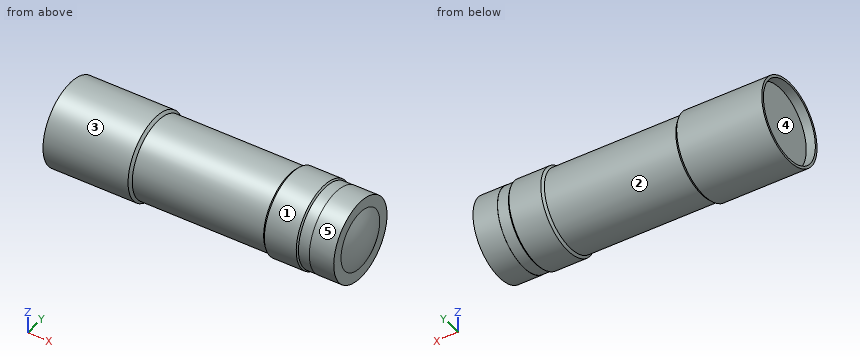
```python
from build123d import *

# Parameters (mm, degrees)
F2_SIZE = 0.74999
F3_SIZE = 0.64999
F4_SIZE = 0.39999


# Not quite as in the source:
# - a fillet or chamfer is up to 0.001 mm smaller than in the source, because OpenCascade refuses the exact size


with BuildPart() as f1:
    # F0 (on Front) → F1 (revolve)
    with BuildSketch(Plane.XZ):
        with BuildLine():
            Line((-85.55, 11.75), (-85.55, 0))
            Line((-85.55, 0), (0, 0))
            ThreePointArc((0, 0), (-0.5715031948, 4.5173277499), (-2.25, 8.75))
            Line((-2.25, 8.75), (-2.25, 12.05))
            Line((-2.25, 12.05), (-9.5, 12.05))
            Line((-9.5, 12.05), (-9.5, 12))
            Line((-9.5, 12), (-12.75, 12))
            Line((-12.75, 12), (-12.75, 12.4))
            Line((-12.75, 12.4), (-23.25, 12.4))
            Line((-23.25, 12.4), (-23.25, 11.75))
            Line((-23.25, 11.75), (-62.25, 11.75))
            Line((-62.25, 11.75), (-62.25, 12.5))
            Line((-62.25, 12.5), (-88.25, 12.5))
            Line((-88.25, 12.5), (-88.25, 11.75))
            Line((-88.25, 11.75), (-85.55, 11.75))
        make_face()
    revolve(axis=Axis((-46.3619604707, 0, 0), (-1, 0, 0)))

    # F2 (size 0.75 in the source; OpenCascade refuses exactly that, so slightly less here)
    f2_edges = [f1.edges().sort_by_distance(p)[0] for p in [
        (-62.25, 0, -12.5),
    ]]
    chamfer(f2_edges, length=F2_SIZE)

    # F3 (size 0.65 in the source; OpenCascade refuses exactly that, so slightly less here)
    f3_edges = [f1.edges().sort_by_distance(p)[0] for p in [
        (-23.25, 0, -12.4),
    ]]
    chamfer(f3_edges, length=F3_SIZE)

    # F4 (size 0.4 in the source; OpenCascade refuses exactly that, so slightly less here)
    f4_edges = [f1.edges().sort_by_distance(p)[0] for p in [
        (-12.75, 0, -12.4),
    ]]
    chamfer(f4_edges, length=F4_SIZE)


solid = f1.part
```
Check sheet for the modelled part. Datum: model origin and axes. Units: mm. Face numbers are marked on the shaded views. A direction names the side the tool comes from. Round coordinates to 2 decimals unless told otherwise and drop trailing zeros. Order: outer loops, then holes, each group sorted by start corner. A loop starts at its lowest first (then second) coordinate and runs counter-clockwise, first axis right, second up. Notation, with made-up numbers: (-32, 39.5) -> (13, 39.5) arc R28 ccw to (13, 69.5) -> close; hole circle Ø2 at (-21.5, 74.25). An arc over 180 degrees is marked (long way). Use CSV: the item, a comma, the result in double quotes.
(1) Tool access check on the marked faces 1, 2 and 3. Record the directions out of +Z, -Z, +X, -X, +Y, -Y that give a thin tool (end or side, any length) a straight path to the whole face; none if there is none.
Worked out:
face 1,"+X"
face 2,"none"
face 3,"+X, -X"
(2) Material ranges on line 1 along Y through (x, z) = (-87.65, 0); line 2 along X through (y, z) = (5, -9.25); line 3 along Z through (x, y) = (-65.5, -1.5), recorded low to high. Write a range as from..to.
Worked out:
line 1,"-12.5..-11.75, 11.75..12.5"
line 2,"-85.55..-2.25"
line 3,"-12.41..12.41"
(3) Depth check by flat-ended pin: pin 1 (5 mm diameter, centred on x = -34, z = 0.5, fed in from +Y); pin 2 (3 mm diameter, centred on x = -44, z = -6, fed in from -Y); pin 3 (1.5 mm diameter, centred on x = -16, z = -2.5, fed in from -Y). Enter the tip coordinate at first touch or a pass-through.
Worked out:
pin 1,"y = 11.75"
pin 2,"y = -10.85"
pin 3,"y = -12.28"
(4) Cross-section at D-D (x = -18). Record the boundary of the cut face in (y, z).
Worked out:
outline,"circle Ø24.8 at (0, 0)"
(5) Draft check along Y on the marked faces 4 and 5. Enter one of: pulls with the +Y half, pulls with the -Y half, needs draft (parallel to the pull), parting line crosses it, or undercut.
Worked out:
face 4,"undercut"
face 5,"parting line crosses it"
(6) Cross-section at C-C (x = -69). Record the boundary of the cut face in (y, z), and give its area (3 significant figures).
Worked out:
outline,"circle Ø25 at (0, 0)"
area,"491 mm²"
